Source: CAD feature listing. Evaluate the final solid. Frame: model axes, mm. Give positions to 0.01 mm unless a question says otherwise; leave off trailing zeros. Loops run counter-clockwise (first coordinate to the right, second up) from the corner with the lowest first, then second, coordinate; pieces in that order, holes last. Notation, with made-up numbers: (61.5, 64) - (69.5, 64) arc R10 cw to (69.5, 76) - close; hole circle Ø1 at (-4, -17). An arc over 180 degrees is marked (long way). Put each result on its own line as item: value.
```python
from build123d import *

# Parameters (mm, degrees)
F1_DEPTH = 12


with BuildPart() as f1:
    # F0 (on Top) → F1 (new body)
    with BuildSketch(Plane.XY):
        with BuildLine():
            Line((152.4, 127), (-152.4, 127))
            Line((-152.4, 127), (-152.4, -88.9))
            ThreePointArc((-152.4, -88.9), (-138.25605, -118.5263), (-106.325581, -126.156122))
            ThreePointArc((-106.325581, -126.156122), (0, -114.904419), (106.325581, -126.156122))
            ThreePointArc((106.325581, -126.156122), (138.25605, -118.5263), (152.4, -88.9))
            Line((152.4, -88.9), (152.4, 127))
        make_face()
    extrude(amount=F1_DEPTH)


solid = f1.part
```
1) Pin query (flat end, axial travel): P1, Ø12, axis at x = -61.5, y = -30.5, coming from the -Z side. Return the tip coordinate at first contact, or that it passes through.
Check result:
P1: z = 0
2) Material intervals for line 1 along Y through (x, z) = (-38.5, 6.25); line 2 along Y through (x, z) = (-21.5, 7.25); line 3 along X through (y, z) = (-102, 3.5), sorted ascending. Write a range as [from, to].
Check result:
line 1: [-116.37, 127]
line 2: [-115.36, 127]
line 3: [-150.08, 150.08]
3) Section query A-A, the plane z = 3. Output: boundary loops of the cut face in (x, y).
Check result:
outline: (-152.4, -88.9) arc R38.1 ccw to (-106.33, -126.16) arc R508 cw to (106.33, -126.16) arc R38.1 ccw to (152.4, -88.9) - (152.4, 127) - (-152.4, 127) - close
4) Section query C-C, the plane y = -110. Output: boundary loops of the cut face in (x, z), plus the area to 3 significant figures.
Check result:
outline: (-146.02, 0) - (146.02, 0) - (146.02, 12) - (-146.02, 12) - close
area: 3,500 mm²
5) Section query B-B, the plane x = 0. Output: boundary loops of the cut face in (y, z), plus the area to 3 significant figures.
Check result:
outline: (-114.9, 0) - (127, 0) - (127, 12) - (-114.9, 12) - close
area: 2,900 mm²
6) Mould query, pull axis X, two halves, no side actions, for faces 1 (the cylindrical face through (-1.5, -114.907, 5.916)), 2 (the flat face through (-2, 2, 12)), 3 (the flat face through (-152.4, 21, 6)), 4 (the flat face through (152.4, 18, 6)). Classes: pulls with the +X half, pulls with the -X half, needs draft (parallel to the pull), parting line crosses it, or undercut.
Check result:
face 1: undercut
face 2: needs draft
face 3: pulls with the -X half
face 4: pulls with the +X half
